from build123d import *

# Parameters (mm, degrees)
SKETCH1_W                  = 76.2
SKETCH1_H                  = 76.2
BOSS_EXTRUDE1_DEPTH        = 12.7
F_10_32_TAPPED_HOLE1_D     = 4.0386
F_10_32_TAPPED_HOLE1_DEPTH = 9.652
F_10_32_TAPPED_HOLE1_TIP   = 1.213317848
SKETCH9_R                  = 25.4
CUT_EXTRUDE2_DEPTH         = 56.358016583
FILLET1_R                  = 38.1


with BuildPart() as part:
    # Sketch1 → Boss-Extrude1 (new body)
    with BuildSketch(Plane(origin=(0, 0, 0), x_dir=(1, 0, 0), z_dir=(0, 1, 0))):
        Rectangle(SKETCH1_W, SKETCH1_H)
    extrude(amount=BOSS_EXTRUDE1_DEPTH)

    # #10-32 Tapped Hole1
    with Locations(Plane(origin=(38.1, 0, 0), x_dir=(0, 0, -1), z_dir=(1, 0, 0))):
        with Locations((-25.4, 6.35), (25.4, 6.35)):
            Hole(F_10_32_TAPPED_HOLE1_D / 2, depth=F_10_32_TAPPED_HOLE1_DEPTH)
            with Locations((0, 0, -(F_10_32_TAPPED_HOLE1_DEPTH + F_10_32_TAPPED_HOLE1_TIP / 2))):  # 118° drill point
                Cone(0, F_10_32_TAPPED_HOLE1_D / 2, F_10_32_TAPPED_HOLE1_TIP, mode=Mode.SUBTRACT)

    # Sketch9 → Cut-Extrude2 (cut, through all)
    with BuildSketch(Plane(origin=(0, 12.7, 0), x_dir=(1, 0, 0), z_dir=(0, 1, 0))):
        with Locations(Location((0, 0, 0), (0, 0, 270))):
            Circle(SKETCH9_R)
    extrude(amount=-CUT_EXTRUDE2_DEPTH, mode=Mode.SUBTRACT)

    # Fillet1
    fillet1_edges = [part.edges().sort_by_distance(p)[0] for p in [
        (-38.1, 6.35, -38.1),
        (-38.1, 6.35, 38.1),
    ]]
    fillet(fillet1_edges, radius=FILLET1_R - 0.0001)  # a hair under: the kernel refuses the full size


solid = part.part
Part model, mm, in its own coordinate system. A direction names the side the tool comes from. Coordinates: 2 decimals unless noted, no trailing zeros. Order: outer loops, then holes, each group sorted by start corner. A loop starts at its lowest first (then second) coordinate and runs counter-clockwise, first axis right, second up. Notation, with made-up numbers: M 31.5,-40 L 50.5,-40 A33 cw 50.5,-2 Z; hole C 60,-38 d5. An arc over 180 degrees is marked long. Use a Markdown table: item, result.
(1) Pull direction Z, two halves, no side cores. Call faces 3 (the flat face through (19, 6, -38.1)), 4 (the cylindrical face through (-15.456, 6.439, -20.157)), 5 (the flat face through (25, 12.7, 8)): released by +Z, released by -Z, zero draft, split by the parting line, or undercut.
A:
| item | result |
|---|---|
| face 3 | released by -Z |
| face 4 | undercut |
| face 5 | zero draft |
(2) Cut at B-B on x = 30. Write the cut outline in (y, z).
A:
| item | result |
|---|---|
| outline | M 0,-38.1 L 12.7,-38.1 L 12.7,38.1 L 0,38.1 Z; hole C 6.35,-25.4 d4.04; hole C 6.35,25.4 d4.04 |
(3) Cut at D-D on x = -18. Write the cut outline in (y, z), then the cut area to 3 significant figures.
A:
| item | result |
|---|---|
| outline | M 0,-33.58 L 12.7,-33.58 L 12.7,-17.92 L 0,-17.92 Z; M 0,17.92 L 12.7,17.92 L 12.7,33.58 L 0,33.58 Z |
| area | 398 mm^2 |
(4) Tool access for faces 1 (the flat face through (25, 0, 8)), 2 (the cylindrical face through (33.206, 6.439, -27.417)): list every direction of +Z, -Z, +X, -X, +Y, -Y with a clear straight run to the whole face (end or side of a thin tool).
A:
| item | result |
|---|---|
| face 1 | +Z, -Z, +X, -X, -Y |
| face 2 | +X |
(5) Flat gauge pins, fed straight in: pin 1 (4.5 mm diameter, centred on y = 6.35, z = -25.4, fed in from +X); pin 2 (3 mm diameter, centred on y = 6.35, z = 25.4, fed in from -X); pin 3 (4 mm diameter, centred on x = -24.5, y = 8, fed in from -Z); pin 4 (6 mm diameter, centred on y = 2, z = 5, fed in from -X). Where does each tip first touch, or does it go through?
A:
| item | result |
|---|---|
| pin 1 | stops at x = 38.1 |
| pin 2 | stops at x = -29.67 |
| pin 3 | stops at z = -30.75 |
| pin 4 | stops at x = -38.05 |
(6) Probe L1, parallel to Z at x = 31, y = 6.35; L2, parallel to X at y = 6.5, z = 1; L3, parallel to Y at x = 33.5, z = -25.4. List the from-to ranges inside material, lowest first.
A:
| item | result |
|---|---|
| L1 | z = -38.1 to -27.42, -23.38 to 23.38, 27.42 to 38.1 |
| L2 | x = -38.09 to -25.38, 25.38 to 38.1 |
| L3 | y = 0 to 4.33, 8.37 to 12.7 |
(7) Cut at C-C on z = 19.5. Write the cut outline in (x, y), then the cut area to 3 significant figures.
A:
| item | result |
|---|---|
| outline | M -32.73,0 L -16.28,0 L -16.28,12.7 L -32.73,12.7 Z; M 16.28,0 L 38.1,0 L 38.1,12.7 L 16.28,12.7 Z |
| area | 486 mm^2 |
